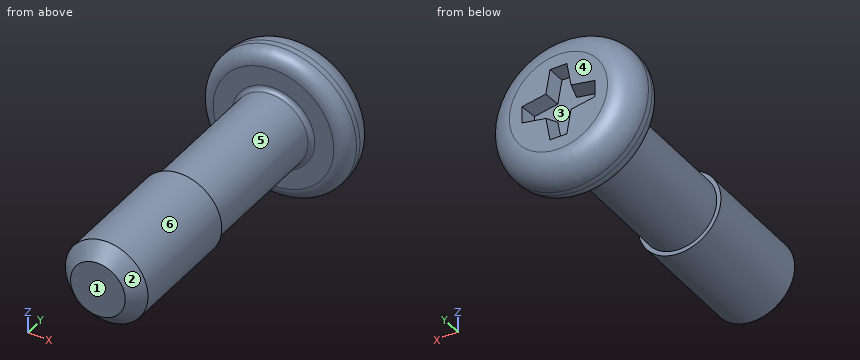
from build123d import *

# Parameters (mm, degrees)
CUT_EXTRUDE1_DEPTH = 0.5
CUT_EXTRUDE1_TAPER = 15


with BuildPart() as part:
    # Sketch1 → Revolve1 (revolve)
    with BuildSketch(Plane.XY):
        with BuildLine():
            Line((0, -11.6), (0.975, -11.6))
            Line((0.975, -11.6), (1.475, -11.1))
            Line((1.475, -11.1), (1.475, -6.9))
            Line((1.475, -6.9), (1.325, -6.9))
            Line((1.325, -6.9), (1.325, -1.75))
            ThreePointArc((1.325, -1.75), (1.368933983, -1.643933983), (1.475, -1.6))
            Line((1.475, -1.6), (2.15, -1.6))
            ThreePointArc((2.15, -1.6), (2.503553391, -1.453553391), (2.65, -1.1))
            Line((2.65, -1.1), (2.65, -0.9))
            ThreePointArc((2.65, -0.9), (2.386396103, -0.263603897), (1.75, 0))
            Line((1.75, 0), (0, 0))
            Line((0, 0), (0, -11.6))
        make_face()
    revolve(axis=Axis((0, 0, 0), (0, -1, 0)))

    # Sketch2 → Cut-Extrude1 (cut)
    with BuildSketch(Plane(origin=(0, 0, 0), x_dir=(1, 0, 0), z_dir=(0, 1, 0))):
        Polygon((-0.300122066, 1.3), (-0.45, 0.45), (-1.3, 0.300122066), (-1.3, -0.300122066), (-0.45, -0.45), (-0.300122066, -1.3), (0.300122066, -1.3), (0.45, -0.45), (1.3, -0.300122066), (1.3, 0.300122066), (0.45, 0.45), (0.300122066, 1.3), align=None)
    extrude(amount=-CUT_EXTRUDE1_DEPTH, taper=CUT_EXTRUDE1_TAPER, mode=Mode.SUBTRACT)


solid = part.part
Geometry check sheet. Reference: the model listing, model coordinates, mm. Face numbers are marked on the shaded views. A direction names the side the tool comes from. Coordinates: 2 decimals unless noted, no trailing zeros. Order: outer loops, then holes, each group sorted by start corner. A loop starts at its lowest first (then second) coordinate and runs counter-clockwise, first axis right, second up. Notation, with made-up numbers: (87, -12.75) -> (130, -12.75) arc R20 cw to (130, 16.25) -> close; hole circle Ø4 at (16.25, -30.75). An arc over 180 degrees is marked (long way). Use a Markdown table: item, result. Add a question column.
1. Cross-section at A-A (y = -9.5). Enter the section's corners in (x, z) (3 decimals).
2. Set-up check for the marked faces 4, 5 and 6: record each of +Z, -Z, +X, -X, +Y, -Y from which the full face is reachable in a straight line by a thin tool's end or side.
3. Mould release check, pull along X, two halves, no side actions. Record for the marked faces 1, 2 and 3: pulls with the +X half, pulls with the -X half, needs draft (parallel to the pull), parting line crosses it, or undercut.
4. Cross-section at B-B (y = -4). Enter the section's corners in (x, z) (3 decimals), and give its area (3 significant figures).
5. Go/stop test with flat-tipped pins: pin 1 Ø1 at (y, z) = (-1.5, 1.5) entering from +X; pin 2 Ø2 at (x, z) = (-2, 0) entering from -Y (3 decimals); pin 3 Ø2 at (y, z) = (-10, 1.5) entering from -X. Record where each tip stops, or that it passes through.
6. Material ranges on L1, parallel to Z at x = 0, y = -2 (3 decimals); L2, parallel to Y at x = -0.5, z = -0.2; L3, parallel to Z at x = 1.55, y = -1, recorded low to high.
Filled sheet:
| question | item | result |
|---|---|---|
| 1 | outline | circle Ø2.95 at (0, 0) |
| 2 | face 4 | +Z, -Z, +X, -X, +Y |
| 2 | face 5 | none |
| 2 | face 6 | -Y |
| 3 | face 1 | needs draft |
| 3 | face 2 | parting line crosses it |
| 3 | face 3 | undercut |
| 4 | outline | circle Ø2.65 at (0, 0) |
| 4 | area | 5.52 mm2 |
| 5 | pin 1 | x = 2.4 |
| 5 | pin 2 | y = -11.575 |
| 5 | pin 3 | x = -1.39 |
| 6 | L1 | -1.325 to 1.325 |
| 6 | L2 | -11.6 to -0.5 |
| 6 | L3 | -2.15 to 2.15 |
